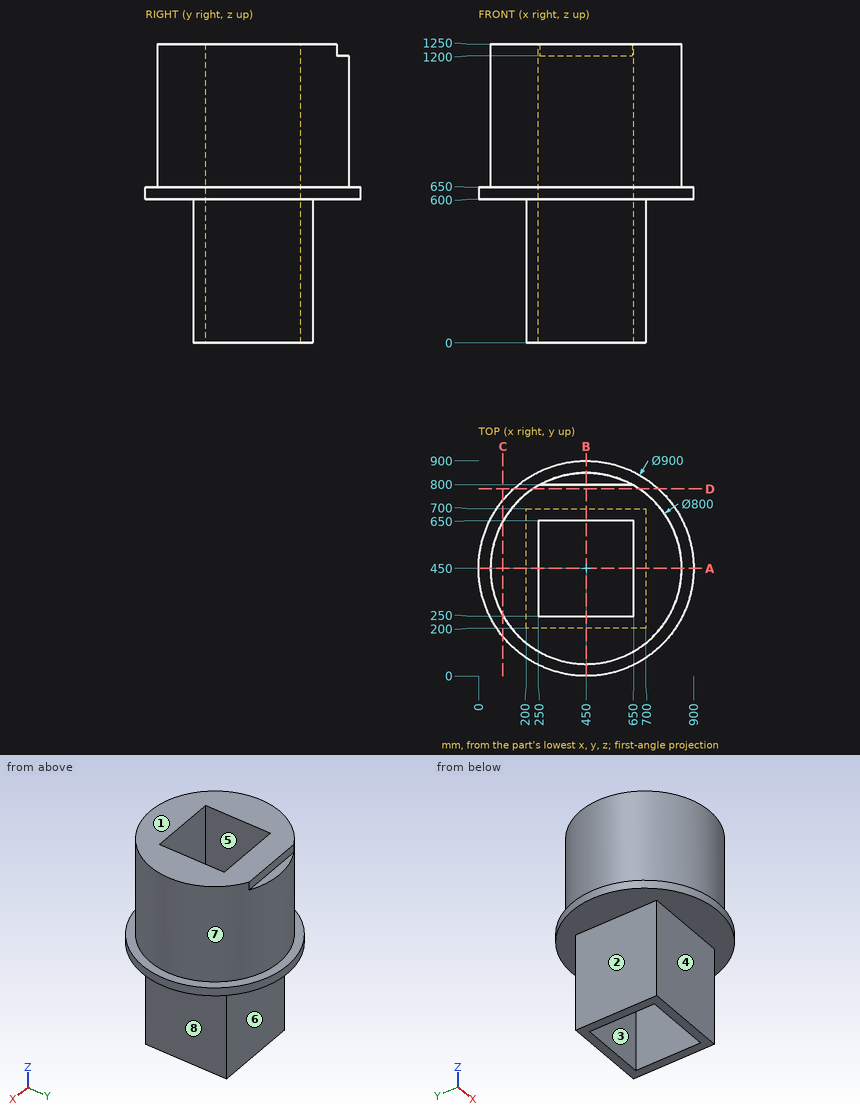
Verification items for this drawing (mm, ordinates from the low corner). A direction names the side the tool comes from. Coordinates: 2 decimals unless noted, no trailing zeros. Loops run counter-clockwise (first coordinate to the right, second up) from the corner with the lowest first, then second, coordinate; pieces in that order, holes last.
Item 1: Sectioned sample at B-B, the plane x = 450. Record the boundary of the cut face in (y, z), then the cut area to 4 significant figures.
Item 2: Access from +Z, -Z, +X, -X, +Y, -Y to the whole of each face (thin tool, end or side, straight path). Record for the marked faces 1, 2, 3 and 4.
Item 3: Sectioned sample at C-C, the plane x = 101.5. Record the boundary of the cut face in (y, z).
Item 4: Go/stop test with flat-tipped pins: pin 1 Ø5 at (x, z) = (238, 368) entering from -Y; pin 2 Ø4 at (x, z) = (564, 953) entering from -Y; pin 3 Ø25 at (x, y) = (384.5, 818.5) entering from +Z. Record where each tip stops, or that it passes through.
Item 5: Sectioned sample at A-A, the plane y = 450. Record the boundary of the cut face in (x, z), then the cut area to 3 significant figures.
Item 6: Sectioned sample at D-D, the plane y = 782.5. Record the boundary of the cut face in (x, z), then the cut area to 3 significant figures.
Item 7: Release check for a two-part mould opening along Y. For the marked faces 5, 6, 7 and 8 record: released by +Y, released by -Y, zero draft, split by the parting line, or undercut.
Item 8: Thickness scan on line 1 (X direction, y = 635, z = 236); line 2 (Z direction, x = 546, y = 782). Record the ranges inside material, lowest first.
Check result:
1. outline: (0, 600) - (200, 600) - (200, 0) - (250, 0) - (250, 1250) - (50, 1250) - (50, 650) - (0, 650) - close; (650, 0) - (700, 0) - (700, 600) - (900, 600) - (900, 650) - (850, 650) - (850, 1200) - (800, 1200) - (800, 1250) - (650, 1250) - close
1. area: 322,500 mm2
2. face 1: +Z, +X, -X, +Y, -Y
2. face 2: -Z, -X, +Y, -Y
2. face 3: +Z, -Z
2. face 4: -Z, +X, -X, -Y
3. outline: (165.31, 600) - (734.69, 600) - (734.69, 650) - (646.34, 650) - (646.34, 1250) - (253.66, 1250) - (253.66, 650) - (165.31, 650) - close
4. pin 1: stops at y = 200
4. pin 2: stops at y = 66
4. pin 3: stops at z = 1200
5. outline: (0, 600) - (200, 600) - (200, 0) - (250, 0) - (250, 1250) - (50, 1250) - (50, 650) - (0, 650) - close; (650, 0) - (700, 0) - (700, 600) - (900, 600) - (900, 650) - (850, 650) - (850, 1250) - (650, 1250) - close
5. area: 325,000 mm2
6. outline: (146.78, 600) - (753.22, 600) - (753.22, 650) - (672.36, 650) - (672.36, 1250) - (227.64, 1250) - (227.64, 650) - (146.78, 650) - close
6. area: 297,000 mm2
7. face 5: undercut
7. face 6: released by +Y
7. face 7: split by the parting line
7. face 8: zero draft
8. line 1: x = 200 to 250, 650 to 700
8. line 2: z = 600 to 1250
